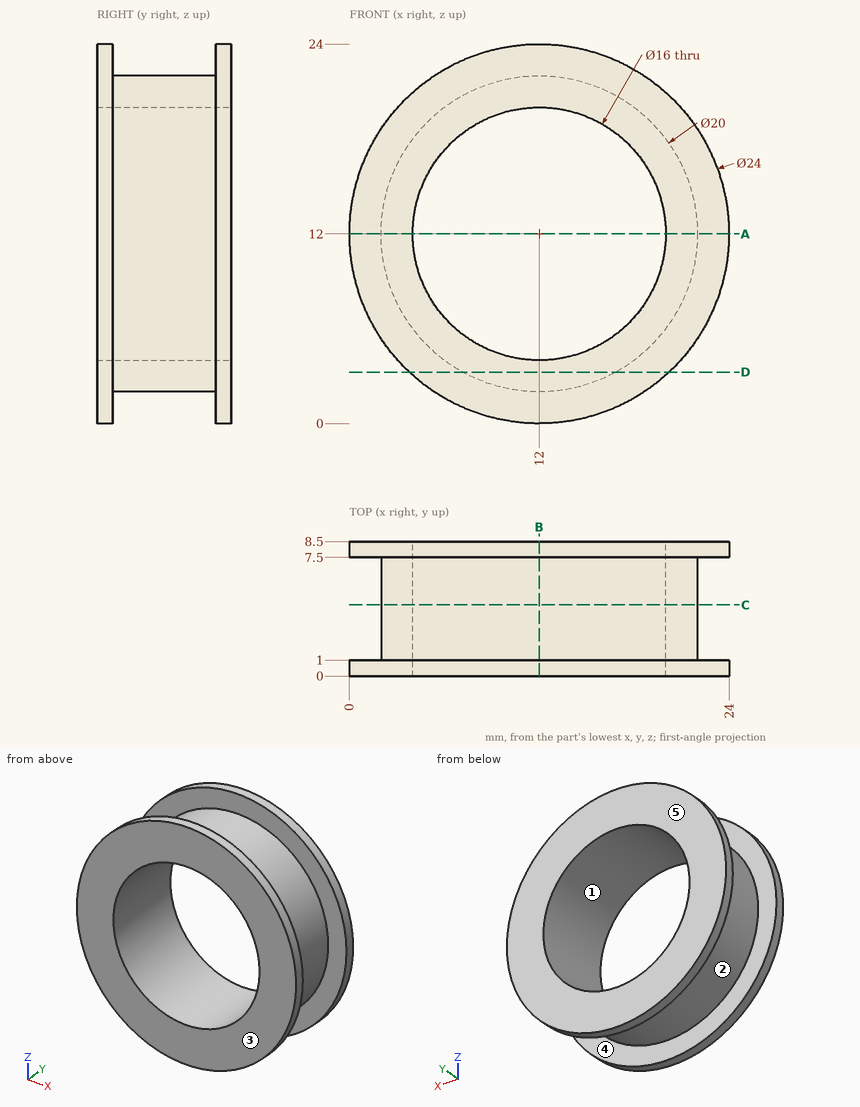
Can you work these out from the drawing? Everything is in mm from the part's minimum corner. A direction names the side the tool comes from. Round coordinates to 2 decimals unless told otherwise and drop trailing zeros. Order: outer loops, then holes, each group sorted by start corner. A loop starts at its lowest first (then second) coordinate and runs counter-clockwise, first axis right, second up.
(1) If we section it at C-C (y = 4.5): Please give me the cut outline in (x, z).
Results are:
outline: circle Ø20 at (12, 12); hole circle Ø16 at (12, 12)
(2) If we section it at D-D (z = 3.25): Please give me the cut outline in (x, y).
Results are:
outline: (3.79, 0) - (20.21, 0) - (20.21, 1) - (16.84, 1) - (16.84, 7.5) - (20.21, 7.5) - (20.21, 8.5) - (3.79, 8.5) - (3.79, 7.5) - (7.16, 7.5) - (7.16, 1) - (3.79, 1) - close
(3) On a 3-axis mill with a long thin cutter (end or side, diameter ignored), from which of +Z, -Z, +X, -X, +Y, -Y can I reach the whole of each face in a straight line? I mean the marked faces 4 and 5. Say none if no direction works.
Results are:
face 4: none
face 5: +Z, -Z, +X, -X, +Y
(4) We'd pull the mould along X, two halves only. Please class the marked faces 1, 2 and 3: +X half, -X half, draft (parallel to the pull), parting line (faces both ways), or undercut.
Results are:
face 1: undercut
face 2: parting line
face 3: draft
(5) If I drill on L1, parallel to Z at x = 12, y = 4; L2, parallel to Y at x = 9.5, z = 1, over which ranges is the centre line in solid material (lowest first)?
Results are:
L1: z = 2 to 4, 20 to 22
L2: y = 0 to 1, 7.5 to 8.5
(6) I'm going to push flat-ended pins straight in: pin 1 (3 mm diameter, centred on x = 8, z = 17, fed in from -Y); pin 2 (1.5 mm diameter, centred on x = 21, y = 6.5, fed in from -Z); pin 3 (12 mm diameter, centred on x = 14, z = 8, fed in from -Y); pin 4 (4 mm diameter, centred on x = 18.5, y = 2, fed in from -Z). Where does each tip first touch, or does it pass through?
Results are:
pin 1: passes through
pin 2: stops at z = 6.35
pin 3: stops at y = 0
pin 4: stops at z = 0.99
(7) If we section it at B-B (x = 12): Please give me the cut outline in (y, z).
Results are:
outline: (0, 0) - (1, 0) - (1, 2) - (7.5, 2) - (7.5, 0) - (8.5, 0) - (8.5, 4) - (0, 4) - close; (0, 20) - (8.5, 20) - (8.5, 24) - (7.5, 24) - (7.5, 22) - (1, 22) - (1, 24) - (0, 24) - close
(8) If we section it at A-A (z = 12): Please give me the cut outline in (x, y).
Results are:
outline: (0, 0) - (4, 0) - (4, 8.5) - (0, 8.5) - (0, 7.5) - (2, 7.5) - (2, 1) - (0, 1) - close; (20, 0) - (24, 0) - (24, 1) - (22, 1) - (22, 7.5) - (24, 7.5) - (24, 8.5) - (20, 8.5) - close
